Design review of the part built by this model. Coordinates are the model's own, in mm. Face numbers are marked on the shaded views. Coordinates: 2 decimals unless noted, no trailing zeros. Loops run counter-clockwise (first coordinate to the right, second up) from the corner with the lowest first, then second, coordinate; pieces in that order, holes last. Notation, with made-up numbers: (-24, -29) - (-4, -29) arc R14 cw to (-4, -6) - close; hole circle Ø2 at (69.25, -2). An arc over 180 degrees is marked (long way). Use one line per item in the form item = value. Start each with the question number.
(1) Clearance check with flat-ended pins moving along their axes: pin 1 Ø6 at (x, z) = (4, -0.5) entering from +Y; pin 2 Ø5 at (y, z) = (14, -5) entering from -X; pin 3 Ø6 at (x, z) = (-2.5, -1) entering from -Y. State where each tip first meets the part, or that it passes through.
(2) For L1, parallel to Z at x = 0, y = 0.2; L2, parallel to Z at x = 3.75, y = 0; L3, parallel to Y at x = -0.75, z = -4, list the stretches that pass through material, from the lowest coordinate up.
(3) Add section B-B (x = 0). State the section outline as (y, z) points, plus the area to 3 significant figures.
(4) The part is to be moulded in two halves that separate along Z. For the marked faces 1, 2 and 3, say which applies: pulls with the +Z half, pulls with the -Z half, needs draft (parallel to the pull), parting line crosses it, or undercut.
(5) Add section A-A (z = 0). State the section outline as (x, y) points, plus the area to 3 significant figures.
(6) Add section D-D (y = 16). State the section outline as (x, z) points, plus the area to 3 significant figures.
(7) Add section C-C (y = 9). State the section outline as (x, z) points.
```python
from build123d import *

# Parameters (mm, degrees)
SKETCH3_R           = 7
BOSS_EXTRUDE1_DEPTH = 2
SKETCH3_3_R         = 7
BOSS_EXTRUDE2_DEPTH = 2
SKETCH5_R           = 6.05
CUT_EXTRUDE1_DEPTH  = 3.2


with BuildPart() as part:
    # Esbo_o1 → Revolu_o1 (revolve)
    with BuildSketch(Plane.XY):
        with BuildLine():
            Line((-6, 0), (0, 0))
            Line((0, 0), (0, 18))
            ThreePointArc((0, 18), (-3.312799908, 15.629316948), (-2.13782919, 11.728775297))
            ThreePointArc((-2.13782919, 11.728775297), (-2.018299709, 11.578229866), (-1.98280027, 11.389309212))
            ThreePointArc((-1.98280027, 11.389309212), (-2.341324967, 8.875429394), (-3.118754256, 6.458047463))
            ThreePointArc((-3.118754256, 6.458047463), (-2.829835487, 5.897588408), (-3.319234982, 5.5))
            Line((-3.319234982, 5.5), (-3.6002073, 5.419432484))
            ThreePointArc((-3.6002073, 5.419432484), (-3.869815727, 4.915531149), (-4.158423427, 4.422265648))
            ThreePointArc((-4.158423427, 4.422265648), (-3.946003212, 3.860595596), (-4.426176527, 3.5))
            Line((-4.426176527, 3.5), (-4.85988246, 3.375636825))
            ThreePointArc((-4.85988246, 3.375636825), (-5.409441117, 2.670828072), (-6, 2))
            Line((-6, 2), (-6, 0))
        make_face()
    revolve(axis=Axis((0, -3.799835873, 0), (0, 1, 0)))

    # Sketch3 → Boss-Extrude1 (add)
    with BuildSketch(Plane.XZ):
        Circle(SKETCH3_R)
    extrude(amount=BOSS_EXTRUDE1_DEPTH)

    # Sketch3_3 → Boss-Extrude2 (add)
    with BuildSketch(Plane.XZ):
        Circle(SKETCH3_3_R)
    extrude(amount=-BOSS_EXTRUDE2_DEPTH)

    # Sketch5 → Cut-Extrude1 (cut)
    with BuildSketch(Plane.XZ.offset(2)):
        Circle(SKETCH5_R)
    extrude(amount=-CUT_EXTRUDE1_DEPTH, mode=Mode.SUBTRACT)


solid = part.part
```
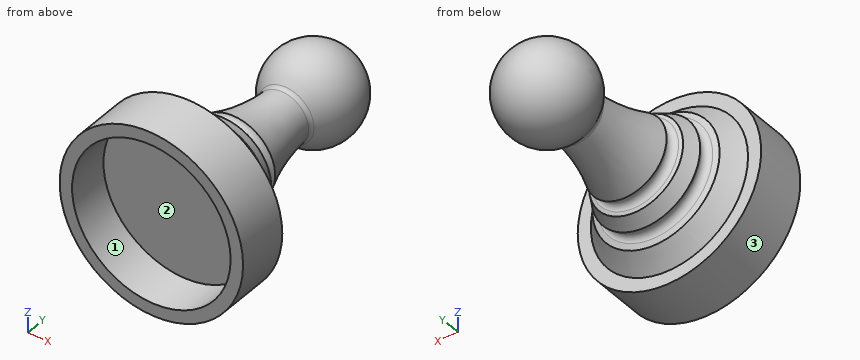
Computed values:
q1.pin_1 = 17.84
q1.pin_2 = -2.42
q1.pin_3 = 1.2
q2.L1 = -7 to -6.05, 6.05 to 7
q2.L2 = -5.91 to -4.75, 4.75 to 5.91
q2.L3 = 1.2 to 3.65, 4.35 to 4.57
q3.outline = (-2, -7) - (2, -7) - (2, -6) arc R15 cw to (3.38, -4.86) - (3.5, -4.43) arc R0.5 cw to (4.42, -4.16) arc R15 cw to (5.42, -3.6) - (5.5, -3.32) arc R0.5 cw to (6.46, -3.12) arc R15 cw to (11.39, -1.98) arc R0.4 cw to (11.73, -2.14) arc R3.5 ccw (long way) to (11.73, 2.14) arc R0.4 cw to (11.39, 1.98) arc R15 cw to (6.46, 3.12) arc R0.5 cw to (5.5, 3.32) - (5.42, 3.6) arc R15 cw to (4.42, 4.16) arc R0.5 cw to (3.5, 4.43) - (3.38, 4.86) arc R15 cw to (2, 6) - (2, 7) - (-2, 7) - (-2, 6.05) - (1.2, 6.05) - (1.2, -6.05) - (-2, -6.05) - close
q3.area = 116 mm^2
q4.face_1 = undercut
q4.face_2 = undercut
q4.face_3 = parting line crosses it
q5.outline = (-7, -2) - (-6.05, -2) - (-6.05, 1.2) - (6.05, 1.2) - (6.05, -2) - (7, -2) - (7, 2) - (6, 2) arc R15 cw to (4.86, 3.38) - (4.43, 3.5) arc R0.5 cw to (4.16, 4.42) arc R15 cw to (3.6, 5.42) - (3.32, 5.5) arc R0.5 cw to (3.12, 6.46) arc R15 cw to (1.98, 11.39) arc R0.4 cw to (2.14, 11.73) arc R3.5 ccw (long way) to (-2.14, 11.73) arc R0.4 cw to (-1.98, 11.39) arc R15 cw to (-3.12, 6.46) arc R0.5 cw to (-3.32, 5.5) - (-3.6, 5.42) arc R15 cw to (-4.16, 4.42) arc R0.5 cw to (-4.43, 3.5) - (-4.86, 3.38) arc R15 cw to (-6, 2) - (-7, 2) - close
q5.area = 116 mm^2
q6.outline = circle Ø6.32 at (0, 0)
q6.area = 31.4 mm^2
q7.outline = circle Ø4.63 at (0, 0)
